The listing builds one solid part. Answer for the finished solid, in the listing's coordinates (mm). Coordinates: 2 decimals unless noted, no trailing zeros. Order: outer loops, then holes, each group sorted by start corner. A loop starts at its lowest first (then second) coordinate and runs counter-clockwise, first axis right, second up. Notation, with made-up numbers: (-3, 65) -> (20, 65) arc R17 cw to (20, 70) -> close; hole circle Ø10 at (47.5, 15.25). An arc over 180 degrees is marked (long way). Write each question's results on one line, items separated by ' | '. Start each with the question number.
(1) Given pin 1 (2 mm diameter, centred on y = -5, z = -26.5, fed in from +X) (3 decimals); pin 2 (5 mm diameter, centred on y = -8, z = -12.5, fed in from -X); pin 3 (4 mm diameter, centred on y = -7.5, z = -21.5, fed in from +X); pin 4 (3 mm diameter, centred on x = -1, y = -9.5, fed in from +Z) (3 decimals), each flat-ended and moving along its own axis, determine where each tip first touches the part or whether it passes through.
(2) Straight lines are drawn through the part: L1, parallel to X at y = -6.5, z = -21.5; L2, parallel to X at y = -6.25, z = -11.5; L3, parallel to Z at x = -1.75, y = -8.25. For each, find the intervals that lie inside material, in ascending order.
(3) The part is cut by section A-A, the plane z = -22.5. Give the vertices of the cut face in (x, y), then the cut area to 3 significant figures.
(4) Determine the mould class of faces 1 (the face through (2.11, -9.39, -39.22)), 2 (the face through (1.14, -9.39, -39.82)), 3 (the face through (0.365, -9.392, -38.648)), 4 (the face through (1.4, 0, -18)) for opening direction X: +X half, -X half, draft (parallel to the pull), parting line (faces both ways), or undercut.
```python
from build123d import *

# Parameters (mm, degrees)
F1_DEPTH    = 19.05
F2_T1_DEPTH = 22.6696744492
F2_T3_DEPTH = 25.3488085544


# Not quite as in the source:
# - a fillet or chamfer that OpenCascade refuses, or shapes differently, is made with other operations: its cross-section is extruded or revolved along the edge and cut away or added


with BuildPart() as f1:
    # F0 (on Front) → F1 (new body)
    with BuildSketch(Plane.XZ):
        with BuildLine():
            ThreePointArc((-1.586615103, -0.0529977822), (-0.0265025846, 1.5872787603), (1.5875, 0))
            ThreePointArc((1.5875, 0), (1.5872787603, -0.0265025846), (1.586615103, -0.0529977822))
            Line((1.586615103, -0.0529977822), (1.4948202515, -2.8010957527))
            ThreePointArc((1.4948202515, -2.8010957527), (2.6951001882, -1.6784099545), (3.173230206, -0.1059955644))
            ThreePointArc((3.173230206, -0.1059955644), (3.1745575207, -0.0530051692), (3.175, 0))
            ThreePointArc((3.175, 0), (-0.0530051692, 3.1745575207), (-3.173230206, -0.1059955644))
            ThreePointArc((-3.173230206, -0.1059955644), (-2.6951001882, -1.6784099545), (-1.4948202515, -2.8010957527))
            Line((-1.4948202515, -2.8010957527), (-1.586615103, -0.0529977822))
        make_face()
        with BuildLine():
            Line((-0.319269794, -37.9940044356), (-1.4948202515, -2.8010957527))
            ThreePointArc((-1.4948202515, -2.8010957527), (-2.6951001882, -1.6784099545), (-3.173230206, -0.1059955644))
            Line((-3.173230206, -0.1059955644), (-1.9976797485, -35.2989042473))
            ThreePointArc((-1.9976797485, -35.2989042473), (-0.7973998118, -36.4215900455), (-0.319269794, -37.9940044356))
        make_face()
        with BuildLine():
            ThreePointArc((3.173230206, -0.1059955644), (2.6951001882, -1.6784099545), (1.4948202515, -2.8010957527))
            Line((1.4948202515, -2.8010957527), (0.319269794, -37.9940044356))
            ThreePointArc((0.319269794, -37.9940044356), (0.7973998118, -36.4215900455), (1.9976797485, -35.2989042473))
            Line((1.9976797485, -35.2989042473), (3.173230206, -0.1059955644))
        make_face()
        with BuildLine():
            ThreePointArc((-0.3175, -38.1), (-0.3179424793, -38.0469948308), (-0.319269794, -37.9940044356))
            ThreePointArc((-0.319269794, -37.9940044356), (-0.7973998118, -36.4215900455), (-1.9976797485, -35.2989042473))
            Line((-1.9976797485, -35.2989042473), (-1.905884897, -38.0470022178))
            ThreePointArc((-1.905884897, -38.0470022178), (-1.9052212397, -38.0734974154), (-1.905, -38.1))
            ThreePointArc((-1.905, -38.1), (-2.0258412421, -38.7075099489), (-2.3699679849, -39.2225320151))
            Line((-2.3699679849, -39.2225320151), (-1.2474359697, -40.3450640303))
            ThreePointArc((-1.2474359697, -40.3450640303), (-0.5591824843, -39.3150198978), (-0.3175, -38.1))
        make_face()
        with BuildLine():
            ThreePointArc((1.9976797485, -35.2989042473), (0.7973998118, -36.4215900455), (0.319269794, -37.9940044356))
            ThreePointArc((0.319269794, -37.9940044356), (0.5393070818, -39.2658801773), (1.2474359697, -40.3450640303))
            Line((1.2474359697, -40.3450640303), (2.3699679849, -39.2225320151))
            ThreePointArc((2.3699679849, -39.2225320151), (2.0159035409, -38.6829400886), (1.905884897, -38.0470022178))
            Line((1.905884897, -38.0470022178), (1.9976797485, -35.2989042473))
        make_face()
    extrude(amount=F1_DEPTH)

    # F2: fillet of radius 0.889 on 4 edges, made by hand

    # F2_s2 → F2_t1 (cut)
    with BuildSketch(Plane.XZ.offset(-1.8098372246)):
        with BuildLine():
            ThreePointArc((-2.0418274273, -38.7447521515), (-2.1035117306, -39.2681046567), (-1.8580687151, -39.7344312849))
            Line((-1.8580687151, -39.7344312849), (-2.3699679849, -39.2225320151))
            ThreePointArc((-2.3699679849, -39.2225320151), (-2.1839076792, -38.9987448959), (-2.0418274273, -38.7447521515))
        make_face()
        with BuildLine():
            ThreePointArc((1.8580687151, -39.7344312849), (2.1035117306, -39.2681046567), (2.0418274273, -38.7447521515))
            ThreePointArc((2.0418274273, -38.7447521515), (2.1839076792, -38.9987448959), (2.3699679849, -39.2225320151))
            Line((2.3699679849, -39.2225320151), (1.8580687151, -39.7344312849))
        make_face()
    extrude(amount=F2_T1_DEPTH, mode=Mode.SUBTRACT)

    # F2_s4 → F2_t3 (cut)
    with BuildSketch(Plane.XZ.offset(-3.1494042772)):
        with BuildLine():
            ThreePointArc((-2.0032929963, -39.5892070037), (-1.1983084283, -39.8319189832), (-0.551076483, -39.2952626045))
            ThreePointArc((-0.551076483, -39.2952626045), (-0.8466666667, -39.8550472849), (-1.2474359697, -40.3450640303))
            Line((-1.2474359697, -40.3450640303), (-2.0032929963, -39.5892070037))
        make_face()
        with BuildLine():
            ThreePointArc((0.551076483, -39.2952626045), (1.1983084283, -39.8319189832), (2.0032929963, -39.5892070037))
            Line((2.0032929963, -39.5892070037), (1.2474359697, -40.3450640303))
            ThreePointArc((1.2474359697, -40.3450640303), (0.8466666667, -39.8550472849), (0.551076483, -39.2952626045))
        make_face()
    extrude(amount=F2_T3_DEPTH, mode=Mode.SUBTRACT)


solid = f1.part
```
Established:
1) pin 1: stops at x = 2.325 | pin 2: stops at x = -2.84 | pin 3: stops at x = 2.53 | pin 4: stops at z = 3.175
2) L1: x = -2.46 to -0.87, 0.87 to 2.46 | L2: x = -2.79 to -1.2, 1.2 to 2.79 | L3: z = -39.77 to 2.65
3) outline: (-2.43, -19.05) -> (-0.84, -19.05) -> (-0.84, 0) -> (-2.43, 0) -> close; (0.84, -19.05) -> (2.43, -19.05) -> (2.43, 0) -> (0.84, 0) -> close | area: 60.5 mm^2
4) face 1: +X half | face 2: undercut | face 3: undercut | face 4: draft
